Read the model definition and answer for the solid it produces. Units are mm, in the model's axes. A direction names the side the tool comes from. Coordinates: 2 decimals unless noted, no trailing zeros. Write each loop counter-clockwise with the first axis right and the second up, starting at its lowest first coordinate (ties: lowest second). Pieces come first, ordered by that corner, then holes.
Item 1: Section B-B (z = -0.25) is taken. Give the vertices of the cut face in (x, y).
Item 2: Determine the mould class of faces 3 (the face through (43.5, 0, 0)), 4 (the face through (-1, 6.35, 0)), 5 (the face through (-19.43, 0.09, 1.07)), 6 (the face through (-36.542, 2.816, 0.111)) for opening direction X: released by +X, released by -X, zero draft, split by the parting line, or undercut.
Item 3: Section C-C (x = -7.02) is taken. Give the vertices of the cut face in (y, z).
Item 4: Straight lines are drawn through the part: probe 1 along Z at (x, y) = (0, 2); probe 2 along X at (y, z) = (1, -5.75); probe 3 along Y at (x, z) = (-38.02, 1.75). For each, find the intervals that lie inside material, in ascending order.
Item 5: This flat-tipped pin is pushed along its axis until it touches: P1, Ø2.5, axis at x = 0, z = 4.63, coming from the -Y side. Where does it stop, or does it pass through?
Item 6: A tool of negligible diameter and unlimited length cuts with its end or side. For faces 1 (the face through (37, -0.35, 0)), 2 (the face through (-1, 0, 7.938)), from which of +Z, -Z, +X, -X, +Y, -Y can it reach the whole face along a straight path? Write none if from no direction.
Item 7: Section A-A (y = 2.35) is taken. State how many separate pieces and enclosed holes the cut face has, then the cut area to 3 significant figures.
Item 8: Section D-D (z = -5.75) is taken. Give the vertices of the cut face in (x, y), then the cut area to 3 significant figures.
from build123d import *

# Parameters (mm, degrees)
SKETCH1_W           = 87
SKETCH1_H           = 12.7
BOSS_EXTRUDE1_DEPTH = 7.9375
SKETCH4_R           = 3
CUT_EXTRUDE2_DEPTH  = 47.005911645
SKETCH2_R           = 1.55
CUT_EXTRUDE1_DEPTH  = 47.739577715
CHAMFER3_SIZE       = 0.5
SKETCH5_R           = 1.375
CUT_EXTRUDE3_DEPTH  = 6
SKETCH6_R           = 1.375
CUT_EXTRUDE4_DEPTH  = 47.005911645


with BuildPart() as part:
    # Sketch1 → Boss-Extrude1 (new, symmetric)
    with BuildSketch(Plane.XY):
        Rectangle(SKETCH1_W, SKETCH1_H)
    extrude(amount=BOSS_EXTRUDE1_DEPTH, both=True)

    # Sketch4 → Cut-Extrude2 (cut, through all)
    with BuildSketch(Plane(origin=(0, 6.35, 0), x_dir=(1, 0, 0), z_dir=(0, 1, 0))):
        with Locations(Location((16.5, -1.7175, 0), (0, 0, 270))):
            Circle(SKETCH4_R)
        with Locations(Location((-16.5, -1.7175, 0), (0, 0, 270))):
            Circle(SKETCH4_R)
    extrude(amount=-CUT_EXTRUDE2_DEPTH, mode=Mode.SUBTRACT)

    # Sketch2 → Cut-Extrude1 (cut, through all)
    with BuildSketch(Plane.XY.offset(7.9375)):
        with Locations((-38.02, 2.35)):
            Circle(SKETCH2_R)
        with Locations((7.02, 2.35)):
            Circle(SKETCH2_R)
        with Locations((-7.02, 2.35)):
            Circle(SKETCH2_R)
        with Locations((38.02, 2.35)):
            Circle(SKETCH2_R)
    extrude(amount=-CUT_EXTRUDE1_DEPTH, mode=Mode.SUBTRACT)

    # Chamfer3
    chamfer3_edges = [part.edges().sort_by_distance(p)[0] for p in [
        (-43.5, 0, 7.9375),
        (0, -6.35, 7.9375),
        (43.5, 0, 7.9375),
        (0, 6.35, 7.9375),
        (43.5, -6.35, 0),
        (-43.5, -6.35, 0),
        (-43.5, 6.35, 0),
        (43.5, 6.35, 0),
    ]]
    chamfer(chamfer3_edges, length=CHAMFER3_SIZE)

    # Sketch5 → Cut-Extrude3 (cut)
    with BuildSketch(Plane(origin=(0, -6.35, 0), x_dir=(1, 0, 0), z_dir=(0, 1, 0))):
        with Locations(Location((-37, 0.3675, 0), (0, 0, 270))):
            Circle(SKETCH5_R)
        with Locations(Location((0, 5.3675, 0), (0, 0, 270))):
            Circle(SKETCH5_R)
        with Locations(Location((37, 0.3675, 0), (0, 0, 90))):
            Circle(SKETCH5_R)
        with Locations(Location((0, -4.6325, 0), (0, 0, 270))):
            Circle(SKETCH5_R)
    extrude(amount=CUT_EXTRUDE3_DEPTH, mode=Mode.SUBTRACT)

    # Sketch6 → Cut-Extrude4 (cut, through all)
    with BuildSketch(Plane.XZ.offset(6.35)):
        with Locations(Location((0, 4.6325, 0), (0, 0, 270))):
            Circle(SKETCH6_R)
        with Locations(Location((0, -5.3675, 0), (0, 0, 270))):
            Circle(SKETCH6_R)
    extrude(amount=-CUT_EXTRUDE4_DEPTH, mode=Mode.SUBTRACT)


solid = part.part
Established:
1. outline: (-43.5, -5.85) - (-43, -6.35) - (-38.37, -6.35) - (-38.37, -0.35) - (-35.63, -0.35) - (-35.63, -6.35) - (-18.76, -6.35) - (-18.76, 6.35) - (-43, 6.35) - (-43.5, 5.85) - close; (-14.24, -6.35) - (14.24, -6.35) - (14.24, 6.35) - (-14.24, 6.35) - close; (18.76, -6.35) - (35.63, -6.35) - (35.63, -0.35) - (38.37, -0.35) - (38.37, -6.35) - (43, -6.35) - (43.5, -5.85) - (43.5, 5.85) - (43, 6.35) - (18.76, 6.35) - close; hole circle Ø3.1 at (-38.02, 2.35); hole circle Ø3.1 at (-7.02, 2.35); hole circle Ø3.1 at (7.02, 2.35); hole circle Ø3.1 at (38.02, 2.35)
2. face 3: released by +X
2. face 4: zero draft
2. face 5: undercut
2. face 6: undercut
3. outline: (-6.35, -7.94) - (0.8, -7.94) - (0.8, 7.94) - (-5.85, 7.94) - (-6.35, 7.44) - close; (3.9, -7.94) - (6.35, -7.94) - (6.35, 7.44) - (5.85, 7.94) - (3.9, 7.94) - close
4. probe 1: z = -7.94 to -6.74, -3.99 to 3.26, 6.01 to 7.94
4. probe 2: x = -43.5 to -38.78, -37.26 to -7.78, -6.26 to -1.32, 1.32 to 6.26, 7.78 to 37.26, 38.78 to 43.5
4. probe 3: y = -6.35 to 0.8, 3.9 to 6.35
5. P1: passes through
6. face 1: -Y
6. face 2: +Z, +X, -X, +Y, -Y
7. separate pieces: 5
7. enclosed holes: 4
7. area: 1,120 mm2
8. outline: (-43.5, -5.85) - (-43, -6.35) - (-1.32, -6.35) - (-1.32, 6.35) - (-43, 6.35) - (-43.5, 5.85) - close; (1.32, -6.35) - (43, -6.35) - (43.5, -5.85) - (43.5, 5.85) - (43, 6.35) - (1.32, 6.35) - close; hole circle Ø3.1 at (-38.02, 2.35); hole circle Ø3.1 at (-7.02, 2.35); hole circle Ø3.1 at (7.02, 2.35); hole circle Ø3.1 at (38.02, 2.35)
8. area: 1,040 mm2
